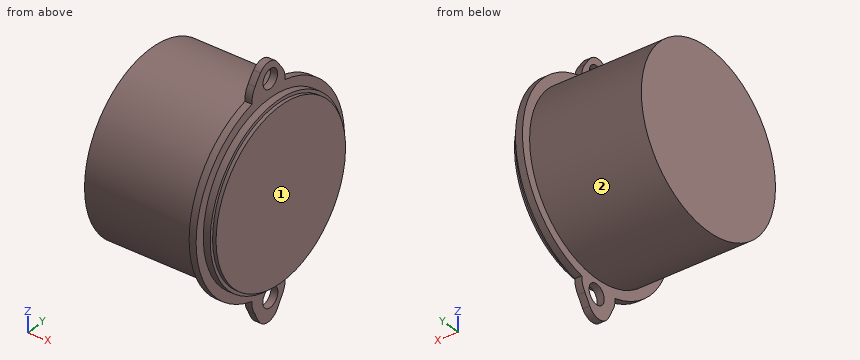
Autodesk Inventor part; units mm, degrees
ref_plane "YZ Plane" through (0, 0, 0) normal (1, 0, 0) x (0, 1, 0)
ref_plane "XZ Plane" through (0, 0, 0) normal (0, 1, 0) x (-1, 0, 0)
ref_plane "XY Plane" through (0, 0, 0) normal (0, 0, 1) x (1, 0, 0)
sketch "Sketch1" plane through (0, 0, 0) normal (1, 0, 0) x (0, 1, 0)
  circle A0 centre (0, 0) radius 12.5
  dimension "d0" = 25
extrude "Extrusion1" add sketch "Sketch1" along normal blind 16
sketch "Sketch2" plane through (16, 0, 0) normal (1, 0, 0) x (0, 0, -1)
  circle A0 centre (0, 0) radius 13.8287
  arc A1 (-13.5463, 2.7804) -> (-13.3988, -3.4214) centre (-13.6396, -0.3245) ccw
  arc A2 (13.3988, -3.4214) -> (13.5463, 2.7804) centre (13.6137, -0.3239) ccw
  line L0 (-15.4609, 2.1919) -> (-18.4894, 0)
  arc A3 (-18.4894, 0) -> (-15.4609, -2.8409) centre (-9.6242, 6.4162) ccw
  line L1 (15.4336, 2.1919) -> (18.879, 0)
  arc A4 (15.4336, -2.8396) -> (18.879, 0) centre (12.797, 3.8693) ccw
extrude "Extrusion2" add sketch "Sketch2" along normal blind 1
fillet "Fillet1" radius 2 2 edges at (16.5, 0, 18.4894) (16.5, 0, -18.879)
sketch "Sketch3" plane through (17, 0, 0) normal (1, 0, 0) x (0, 0, -1)
  circle A0 centre (0, 0) radius 12.5
extrude "Extrusion3" add sketch "Sketch3" along normal blind 1
sketch "Sketch4" plane through (17, 0, 0) normal (1, 0, 0) x (0, 0, -1)
  circle A0 centre (-15.0948, 0) radius 1.3586
  circle A1 centre (14.6009, 0) radius 1.4082
  point P0 (0, 0)
extrude "Extrusion4" cut sketch "Sketch4" against normal blind 1
sketch "Sketch5" plane through (18, 0, 0) normal (1, 0, 0) x (0, 0, -1)
  point P0 (0, 0)
sketch "Sketch6" plane through (18, 0, 0) normal (1, 0, 0) x (0, 0, -1)
  circle A0 centre (0, 0) radius 12.0611
extrude "Extrusion5" add sketch "Sketch6" along normal blind 0.5
properties part number "PIEZO"
CAD build for the part. Positions are in the model's coordinates, mm. Face numbers are marked on the shaded views. A direction names the side the tool comes from. Give positions to 0.01 mm unless a question says otherwise; leave off trailing zeros. Write each loop counter-clockwise with the first axis right and the second up, starting at its lowest first coordinate (ties: lowest second). Pieces come first, ordered by that corner, then holes. Notation, with made-up numbers: M 51.5,63 L 80.5,63 A22 ccw 80.5,90 Z; hole C -10,82 d9. An arc over 180 degrees is marked long. Put each result on its own line as item: value. Start each with the question number.
(1) Band-saw the part on D-D, the plane x = 13.5. Write the cut outline in (y, z).
(2) Which spindle directions (+Z, -Z, +X, -X, +Y, -Y) get a long thin tool onto all of the face, cutting with end or side? Do the marked faces 1 and 2. Say none if no direction does.
(3) Band-saw the part on A-A, the plane y = 0. Write the cut outline in (x, z).
(4) Flat gauge pins, fed straight in: pin 1 Ø3.5 at (y, z) = (0, -14.6) entering from -X; pin 2 Ø1.5 at (x, z) = (2.5, -4.5) entering from -Y; pin 3 Ø10 at (x, y) = (3, 9.5) entering from -Z; pin 4 Ø1.6 at (y, z) = (0, 15.09) entering from -X. Where does each tip first touch, or does it go through?
(5) Probe L1, parallel to X at y = -8.5, z = 10; L2, parallel to Y at x = 10.25, z = 2; L3, parallel to Y at x = 4, z = -9.5. List the from-to ranges inside material, lowest first.
(6) Band-saw the part on B-B, the plane z = 0. Write the cut outline in (x, y).
(7) Band-saw the part on C-C, the plane y = -9.75. Write the cut outline in (x, z), and give its area (3 significant figures).
Response values:
1. outline: C 0,0 d25
2. face 1: +Z, -Z, +X, +Y, -Y
2. face 2: -X
3. outline: M 0,-12.5 L 16,-12.5 L 16,-13.19 L 17,-13.19 L 17,-12.5 L 18,-12.5 L 18,-12.06 L 18.5,-12.06 L 18.5,12.06 L 18,12.06 L 18,12.5 L 17,12.5 L 17,13.74 L 16,13.74 L 16,12.5 L 0,12.5 Z; M 16,-17.74 L 17,-17.74 L 17,-16.01 L 16,-16.01 Z; M 16,16.45 L 17,16.45 L 17,17.49 L 16,17.49 Z
4. pin 1: stops at x = 16
4. pin 2: stops at y = -11.92
4. pin 3: stops at z = -11.66
4. pin 4: passes through
5. L1: x = 16 to 17
5. L2: y = -12.34 to 12.34
5. L3: y = -8.12 to 8.12
6. outline: M 0,-12.5 L 16,-12.5 L 16,-13.83 L 17,-13.83 L 17,-12.5 L 18,-12.5 L 18,-12.06 L 18.5,-12.06 L 18.5,12.06 L 18,12.06 L 18,12.5 L 17,12.5 L 17,13.83 L 16,13.83 L 16,12.5 L 0,12.5 Z
7. outline: M 0,-7.82 L 16,-7.82 L 16,-9.81 L 17,-9.81 L 17,-7.82 L 18,-7.82 L 18,-7.1 L 18.5,-7.1 L 18.5,7.1 L 18,7.1 L 18,7.82 L 17,7.82 L 17,9.81 L 16,9.81 L 16,7.82 L 0,7.82 Z
7. area: 293 mm2
